Geometry check sheet. Reference: the model listing, model coordinates, mm. A direction names the side the tool comes from. Round coordinates to 2 decimals unless told otherwise and drop trailing zeros. Write each loop counter-clockwise with the first axis right and the second up, starting at its lowest first coordinate (ties: lowest second). Pieces come first, ordered by that corner, then holes. Notation, with made-up numbers: M 31.25,88 L 90.25,88 A32 cw 90.25,121 Z; hole C 71,58 d5. An arc over 180 degrees is marked long. Answer in a Markdown table with one row per item. Add a question column.
from build123d import *

# Parameters (mm, degrees)
SKIZZE1_W                                            = 216
SKIZZE1_H                                            = 100
AUFSATZ_LINEAR_AUSTRAGEN1_DEPTH                      = 10
STIRNSENKUNG_F_R_M6_ZYLINDERSCHRAUBE_MIT_D           = 6.6
STIRNSENKUNG_F_R_M6_ZYLINDERSCHRAUBE_MIT_DEPTH       = 15
STIRNSENKUNG_F_R_M6_ZYLINDERSCHRAUBE_MIT_CBORE_D     = 11
STIRNSENKUNG_F_R_M6_ZYLINDERSCHRAUBE_MIT_CBORE_DEPTH = 6.4
STIRNSENKUNG_F_R_M6_ZYLINDERSCHRAUBE_MIT_TIP         = 1.982840043
CBORE_FOR_M6_HEX_SOCKET_HEAD_CAP_SCREW1_D            = 6.6
CBORE_FOR_M6_HEX_SOCKET_HEAD_CAP_SCREW1_DEPTH        = 15
CBORE_FOR_M6_HEX_SOCKET_HEAD_CAP_SCREW1_CBORE_D      = 11
CBORE_FOR_M6_HEX_SOCKET_HEAD_CAP_SCREW1_CBORE_DEPTH  = 6.4
CBORE_FOR_M6_HEX_SOCKET_HEAD_CAP_SCREW1_TIP          = 1.982840043
M8_CLEARANCE_HOLE1_D                                 = 8.4
M8_CLEARANCE_HOLE1_DEPTH                             = 17
M8_CLEARANCE_HOLE1_TIP                               = 2.5236146
SKIZZE18_W                                           = 54
SKIZZE18_H                                           = 26
SCHNITT_LINEAR_AUSTRAGEN1_DEPTH                      = 15
SKETCH1_W                                            = 27
SKETCH1_H                                            = 10
BOSS_EXTRUDE1_DEPTH                                  = 9.5
CUT_EXTRUDE1_DEPTH                                   = 10
LPATTERN1_COUNT                                      = 2
LPATTERN1_PITCH                                      = 19
CUT_EXTRUDE2_START                                   = -10
CUT_EXTRUDE2_DEPTH                                   = 3
LPATTERN2_COUNT                                      = 2
LPATTERN2_PITCH                                      = 19
MIRROR1_COPY_1_DEPTH                                 = 10
MIRROR1_START                                        = -10
MIRROR1_COPY_2_DEPTH                                 = 3
SKETCH5_W                                            = 27
SKETCH5_H                                            = 9.5
CUT_EXTRUDE3_DEPTH                                   = 10
CHAMFER4_SIZE                                        = 3
CHAMFER5_SIZE                                        = 3


with BuildPart() as part:
    # Skizze1 → Aufsatz-Linear austragen1 (new body)
    with BuildSketch(Plane.XY):
        Rectangle(SKIZZE1_W, SKIZZE1_H)
    extrude(amount=AUFSATZ_LINEAR_AUSTRAGEN1_DEPTH)

    # Stirnsenkung für M6 Zylinderschraube mit Innensechskant1
    with Locations(Plane.XY.offset(10)):
        with Locations((-47, -43.5), (47, -43.5)):
            CounterBoreHole(STIRNSENKUNG_F_R_M6_ZYLINDERSCHRAUBE_MIT_D / 2, STIRNSENKUNG_F_R_M6_ZYLINDERSCHRAUBE_MIT_CBORE_D / 2, STIRNSENKUNG_F_R_M6_ZYLINDERSCHRAUBE_MIT_CBORE_DEPTH, depth=STIRNSENKUNG_F_R_M6_ZYLINDERSCHRAUBE_MIT_DEPTH)
            with Locations((0, 0, -(STIRNSENKUNG_F_R_M6_ZYLINDERSCHRAUBE_MIT_DEPTH + STIRNSENKUNG_F_R_M6_ZYLINDERSCHRAUBE_MIT_TIP / 2))):  # 118° drill point
                Cone(0, STIRNSENKUNG_F_R_M6_ZYLINDERSCHRAUBE_MIT_D / 2, STIRNSENKUNG_F_R_M6_ZYLINDERSCHRAUBE_MIT_TIP, mode=Mode.SUBTRACT)

    # CBORE for M6 Hex Socket Head Cap Screw1
    with Locations(Plane.XY.offset(10)):
        with Locations((-47, 43.5), (47, 43.5)):
            CounterBoreHole(CBORE_FOR_M6_HEX_SOCKET_HEAD_CAP_SCREW1_D / 2, CBORE_FOR_M6_HEX_SOCKET_HEAD_CAP_SCREW1_CBORE_D / 2, CBORE_FOR_M6_HEX_SOCKET_HEAD_CAP_SCREW1_CBORE_DEPTH, depth=CBORE_FOR_M6_HEX_SOCKET_HEAD_CAP_SCREW1_DEPTH)
            with Locations((0, 0, -(CBORE_FOR_M6_HEX_SOCKET_HEAD_CAP_SCREW1_DEPTH + CBORE_FOR_M6_HEX_SOCKET_HEAD_CAP_SCREW1_TIP / 2))):  # 118° drill point
                Cone(0, CBORE_FOR_M6_HEX_SOCKET_HEAD_CAP_SCREW1_D / 2, CBORE_FOR_M6_HEX_SOCKET_HEAD_CAP_SCREW1_TIP, mode=Mode.SUBTRACT)

    # M8 Clearance Hole1
    with Locations(Plane.XY.offset(10)):
        with Locations((-101, 17), (-101, -43), (101, 17), (101, -43)):
            Hole(M8_CLEARANCE_HOLE1_D / 2, depth=M8_CLEARANCE_HOLE1_DEPTH)
            with Locations((0, 0, -(M8_CLEARANCE_HOLE1_DEPTH + M8_CLEARANCE_HOLE1_TIP / 2))):  # 118° drill point
                Cone(0, M8_CLEARANCE_HOLE1_D / 2, M8_CLEARANCE_HOLE1_TIP, mode=Mode.SUBTRACT)

    # Skizze18 → Schnitt-Linear austragen1 (cut)
    with BuildSketch(Plane.XY.offset(10)):
        with Locations((-81, 37)):
            Rectangle(SKIZZE18_W, SKIZZE18_H)
    schnitt_linear_austragen1 = extrude(amount=-SCHNITT_LINEAR_AUSTRAGEN1_DEPTH, mode=Mode.SUBTRACT)

    # Spiegeln1: Schnitt-Linear austragen1 across plane
    add(schnitt_linear_austragen1.mirror(Plane(origin=(0, 0, 0), x_dir=(0, 0, 1), z_dir=(1, 0, 0))), mode=Mode.SUBTRACT)

    # Sketch1 → Boss-Extrude1 (add)
    with BuildSketch(Plane(origin=(0, 24, 0), x_dir=(1, 0, 0), z_dir=(0, 1, 0))):
        with Locations((83.5, -5)):
            Rectangle(SKETCH1_W, SKETCH1_H)
    boss_extrude1 = extrude(amount=BOSS_EXTRUDE1_DEPTH)

    # Sketch3 → Cut-Extrude1 (cut)
    with BuildSketch(Plane(origin=(0, 0, 0), x_dir=(-1, 0, 0), z_dir=(0, 0, -1))):
        with BuildLine():
            Line((-91.25, 29.15), (-91.25, 27.35))
            ThreePointArc((-91.25, 27.35), (-93, 25.6), (-94.75, 27.35))
            Line((-94.75, 27.35), (-94.75, 29.15))
            ThreePointArc((-94.75, 29.15), (-93, 30.9), (-91.25, 29.15))
        make_face()
    cut_extrude1 = extrude(amount=-CUT_EXTRUDE1_DEPTH, mode=Mode.SUBTRACT)

    # LPattern1: Cut-Extrude1 ×2
    with Locations(*[(-i * LPATTERN1_PITCH, 0, 0) for i in range(1, LPATTERN1_COUNT)]):
        add(cut_extrude1, mode=Mode.SUBTRACT)

    # Sketch4 → Cut-Extrude2 (cut)
    with BuildSketch(Plane.XY.offset(10).offset(CUT_EXTRUDE2_START)):
        Polygon((74, 32.383161507), (71.2, 30.766580754), (71.2, 28.375279034), (71.2, 25.733419246), (74, 24.116838493), (76.8, 25.733419246), (76.8, 28.372780006), (76.8, 30.766580754), align=None)
    cut_extrude2 = extrude(amount=CUT_EXTRUDE2_DEPTH, mode=Mode.SUBTRACT)

    # LPattern2: Cut-Extrude2 ×2
    with Locations(*[(i * LPATTERN2_PITCH, 0, 0) for i in range(1, LPATTERN2_COUNT)]):
        add(cut_extrude2, mode=Mode.SUBTRACT)

    # Mirror1: Boss-Extrude1, Cut-Extrude1, Cut-Extrude2 across plane
    add(boss_extrude1.mirror(Plane.ZX.offset(-13)))
    add(cut_extrude1.mirror(Plane.ZX.offset(-13)), mode=Mode.SUBTRACT)
    add(cut_extrude2.mirror(Plane.ZX.offset(-13)), mode=Mode.SUBTRACT)

    # Mirror1 copy 1 sketch → Mirror1 copy 1 (cut)
    with BuildSketch(Plane(origin=(-19, -26, 0), x_dir=(-1, 0, 0), z_dir=(0, 0, -1))):
        with BuildLine():
            Line((-91.25, -29.15), (-91.25, -27.35))
            ThreePointArc((-91.25, -27.35), (-93, -25.6), (-94.75, -27.35))
            Line((-94.75, -27.35), (-94.75, -29.15))
            ThreePointArc((-94.75, -29.15), (-93, -30.9), (-91.25, -29.15))
        make_face()
    extrude(amount=-MIRROR1_COPY_1_DEPTH, mode=Mode.SUBTRACT)

    # Mirror1 copy 2 sketch → Mirror1 copy 2 (cut)
    with BuildSketch(Plane(origin=(19, -26, 10), x_dir=(1, 0, 0), z_dir=(0, 0, 1)).offset(MIRROR1_START)):
        Polygon((74, -32.383161507), (71.2, -30.766580754), (71.2, -28.375279034), (71.2, -25.733419246), (74, -24.116838493), (76.8, -25.733419246), (76.8, -28.372780006), (76.8, -30.766580754), align=None)
    extrude(amount=MIRROR1_COPY_2_DEPTH, mode=Mode.SUBTRACT)

    # Sketch5 → Cut-Extrude3 (cut)
    with BuildSketch(Plane.XY.offset(10)):
        with Locations((83.5, 28.75)):
            Rectangle(SKETCH5_W, SKETCH5_H)
    extrude(amount=-CUT_EXTRUDE3_DEPTH, mode=Mode.SUBTRACT)

    # Chamfer4
    chamfer4_edges = [part.edges().sort_by_distance(p)[0] for p in [
        (97, -59.5, 5),
        (70, -59.5, 5),
        (97, -50, 5),
        (70, -50, 5),
        (-54, 24, 5),
        (54, 24, 5),
    ]]
    chamfer(chamfer4_edges, length=CHAMFER4_SIZE)

    # Chamfer5
    chamfer5_edges = [part.edges().sort_by_distance(p)[0] for p in [
        (108, -50, 5),
        (-108, 24, 5),
        (-108, -50, 5),
        (-54, 50, 5),
        (108, 24, 5),
        (54, 50, 5),
    ]]
    chamfer(chamfer5_edges, length=CHAMFER5_SIZE)


solid = part.part
Item 1: Section check A-A, the plane y = 43.5. Record the boundary of the cut face in (x, z), and give its area (3 significant figures).
Item 2: Gauge pin test, flat ends, axial feed: pin 1 Ø2.5 at (y, z) = (-54, 1) entering from -X; pin 2 Ø3.5 at (y, z) = (-55, 1.5) entering from +X; pin 3 Ø0.9 at (y, z) = (-54, 5) entering from -X; pin 4 Ø4 at (x, y) = (-47, -43.5) entering from -Z. Record the tip position at first contact, or that the pin passes through.
Item 3: Section check C-C, the plane y = 17. Record the boundary of the cut face in (x, z).
Item 4: Scan lines: probe 1 along Y at (x, z) = (47, 0.9); probe 2 along Y at (x, z) = (-101, 4.5); probe 3 along X at (y, z) = (-40, 9). Record each from-to range of solid material in increasing order. Write a range as from..to.
Item 5: Access from +Z, -Z, +X, -X, +Y, -Y to the whole of each face (thin tool, end or side, straight path). Record for faces 1 (the flat face through (-81, 24, 5)), 2 (the flat face through (-47, -47, 3.6)), 3 (the cylindrical face through (-103.26, -39.46, 4.93)).
Item 6: Mould release check, pull along X, two halves, no side actions. Record for faces 4 (the flat face through (-54, 37, 5)), 5 (the flat face through (102, -50, 5)), 6 (the flat face through (91, -54, 3)): +X half, -X half, draft (parallel to the pull), parting line (faces both ways), or undercut.
Item 7: Section check D-D, the plane z = 8.25. Give the number of separate pieces and of enclosed holes in the cut face, and give its area (3 significant figures).
Item 8: Section check B-B, the plane x = 47. Record the boundary of the cut face in (y, z), and give its area (3 significant figures).
Result sheet:
| question | item | result |
|---|---|---|
| 1 | outline | M -54,0 L -50.3,0 L -50.3,3.6 L -52.5,3.6 L -52.5,10 L -54,10 Z; M -43.7,0 L 43.7,0 L 43.7,3.6 L 41.5,3.6 L 41.5,10 L -41.5,10 L -41.5,3.6 L -43.7,3.6 Z; M 50.3,0 L 54,0 L 54,10 L 52.5,10 L 52.5,3.6 L 50.3,3.6 Z |
| 1 | area | 892 mm^2 |
| 2 | pin 1 | stops at x = 69.75 |
| 2 | pin 2 | stops at x = 97 |
| 2 | pin 3 | stops at x = 70 |
| 2 | pin 4 | passes through |
| 3 | outline | M -108,0 L -105.2,0 L -105.2,10 L -108,10 Z; M -96.8,0 L 96.8,0 L 96.8,10 L -96.8,10 Z; M 105.2,0 L 108,0 L 108,10 L 105.2,10 Z |
| 4 | probe 1 | y = -50..-46.8, -40.2..40.2, 46.8..50 |
| 4 | probe 2 | y = -50..-47.2, -38.8..12.8, 21.2..24 |
| 4 | probe 3 | x = -108..-103.94, -98.06..-51.24, -42.76..42.76, 51.24..98.06, 103.94..108 |
| 5 | face 1 | +Z, -Z, -X, +Y |
| 5 | face 2 | +Z |
| 5 | face 3 | +Z, -Z |
| 6 | face 4 | -X half |
| 6 | face 5 | draft |
| 6 | face 6 | undercut |
| 7 | separate pieces | 1 |
| 7 | enclosed holes | 10 |
| 7 | area | 18,400 mm^2 |
| 8 | outline | M -50,0 L -46.8,0 L -46.8,3.6 L -49,3.6 L -49,10 L -50,10 Z; M -40.2,0 L 40.2,0 L 40.2,3.6 L 38,3.6 L 38,10 L -38,10 L -38,3.6 L -40.2,3.6 Z; M 46.8,0 L 50,0 L 50,10 L 49,10 L 49,3.6 L 46.8,3.6 Z |
| 8 | area | 812 mm^2 |
